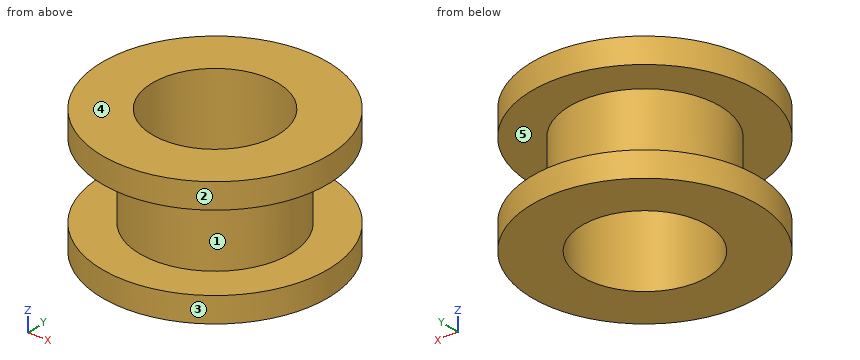
```python
from build123d import *

# Parameters (mm, degrees)
SKETCH_1_R      = 9
SKETCH_1_R_2    = 5
EXTRUDE_1_DEPTH = 2
SKETCH_2_R      = 6
SKETCH_2_R_2    = 5
EXTRUDE_2_DEPTH = 8
EXTRUDE_START   = -2
SKETCH_3_R      = 9
SKETCH_3_R_2    = 5
EXTRUDE_3_DEPTH = 2


with BuildPart() as part:
    # 草图1 → 凸台-拉伸1 (new body)
    with BuildSketch(Plane.XY):
        with Locations((0, 118.25)):
            Circle(SKETCH_1_R)
        with Locations((0, 118.25)):
            Circle(SKETCH_1_R_2, mode=Mode.SUBTRACT)
    extrude(amount=EXTRUDE_1_DEPTH)

    # 草图2 → 凸台-拉伸2 (add)
    with BuildSketch(Plane.XY.offset(2)):
        with Locations(Location((0, 118.25, 0), (0, 0, 180))):
            Circle(SKETCH_2_R)
        with Locations(Location((0, 118.25, 0), (0, 0, 180))):
            Circle(SKETCH_2_R_2, mode=Mode.SUBTRACT)
    extrude(amount=EXTRUDE_2_DEPTH)

    # 草图3 → 凸台-拉伸3 (add)
    with BuildSketch(Plane.XY.offset(10).offset(EXTRUDE_START)):
        with Locations((0, 118.25)):
            Circle(SKETCH_3_R)
        with Locations(Location((0, 118.25, 0), (0, 0, 180))):
            Circle(SKETCH_3_R_2, mode=Mode.SUBTRACT)
    extrude(amount=EXTRUDE_3_DEPTH)


solid = part.part
```
Build history of the part. All positions in model axes, mm. Face numbers are marked on the shaded views. A direction names the side the tool comes from. Coordinates: 2 decimals unless noted, no trailing zeros. Write each loop counter-clockwise with the first axis right and the second up, starting at its lowest first coordinate (ties: lowest second). Pieces come first, ordered by that corner, then holes.
1. Band-saw the part on C-C, the plane z = 7.25. Give the cut face in (x, y), and give its area (3 significant figures).
Answer block:
outline: circle Ø12 at (0, 118.25); hole circle Ø10 at (0, 118.25)
area: 34.6 mm2
2. Band-saw the part on A-A, the plane y = 113.5. Give the cut face in (x, z).
Answer block:
outline: (-7.64, 0) - (-1.56, 0) - (-1.56, 10) - (-7.64, 10) - (-7.64, 8) - (-3.67, 8) - (-3.67, 2) - (-7.64, 2) - close; (1.56, 0) - (7.64, 0) - (7.64, 2) - (3.67, 2) - (3.67, 8) - (7.64, 8) - (7.64, 10) - (1.56, 10) - close
3. Pull direction Z, two halves, no side cores. Call the marked faces 3, 4 and 5: released by +Z, released by -Z, zero draft, split by the parting line, or undercut.
Answer block:
face 3: zero draft
face 4: released by +Z
face 5: undercut
4. Band-saw the part on D-D, the plane y = 111.5. Give the cut face in (x, z), and give its area (3 significant figures).
Answer block:
outline: (-5.95, 0) - (5.95, 0) - (5.95, 2) - (-5.95, 2) - close; (-5.95, 8) - (5.95, 8) - (5.95, 10) - (-5.95, 10) - close
area: 47.6 mm2
5. 3-axis set-ups, long thin cutter, end or side, ignore diameter. For the marked faces 1 and 2: which of +Z, -Z, +X, -X, +Y, -Y reach the whole face in a straight line?
Answer block:
face 1: none
face 2: +Z, -Z
6. Drop flat-ended pins along their axis: pin 1 (5 mm diameter, centred on y = 121, z = 2.5, fed in from +X) (3 decimals); pin 2 (5 mm diameter, centred on x = -1.5, z = 5, fed in from -Y). Give the stop position or say it passes through.
Answer block:
pin 1: stops at x = 8.995
pin 2: stops at y = 112.25
7. Drill centre lines: probe 1 along Z at (x, y) = (-7.5, 122.75); probe 2 along Y at (x, z) = (0, 2.75); probe 3 along X at (y, z) = (118.25, 3.5). Where is each one in solid material? Low to high.
Answer block:
probe 1: z = 0 to 2, 8 to 10
probe 2: y = 112.25 to 113.25, 123.25 to 124.25
probe 3: x = -6 to -5, 5 to 6
